from build123d import *

# Parameters (mm, degrees)
F0_T = -12.7
F1_R = 5.08


with BuildPart() as f3:
    # F2 (on Front) → F3 (revolve)
    with BuildSketch(Plane.XZ):
        Polygon((42.4395352602, 50.6010726094), (0, 50.6010726094), (0, -51.2385219336), (24.419054389, -51.2385219336), align=None)
    revolve(axis=Axis((0, 0, -0.3187246621), (0, 0, 1)))

    # F0
    f0_openings = [f3.faces().sort_by_distance(p)[0] for p in [
        (0, 0, 50.601073),
    ]]
    offset(amount=F0_T, openings=f0_openings)

    # F1
    f1_edges = [f3.edges().sort_by_distance(p)[0] for p in [
        (-42.439535, 0, 50.601073),
        (-29.542242, 0, 50.601073),
    ]]
    fillet(f1_edges, radius=F1_R)


solid = f3.part
Here's how the part is built. I have some questions about the finished solid (model axes, mm). Round coordinates to 2 decimals unless told otherwise and drop trailing zeros. Loops run counter-clockwise (first coordinate to the right, second up) from the corner with the lowest first, then second, coordinate; pieces in that order, holes last.
1. If we section it at D-D on z = -45: Write out the boundary of the cut face in (x, y).
Answer list:
outline: circle Ø51.05 at (0, 0)
2. If I drill on line 1 along Z through (x, y) = (-8, 0.5); line 2 along Y through (x, z) = (18.5, 37); line 3 along Y through (x, z) = (14.5, 17.5), over which ranges is the centre line in solid material (lowest first)?
Answer list:
line 1: z = -51.24 to -38.54
line 2: y = -35.5 to -19.85, 19.85 to 35.5
line 3: y = -33.59 to -18.73, 18.73 to 33.59
3. We'd pull the mould along Y, two halves only. Please class faces 1 (the face through (0, 0, -38.539)), 2 (the face through (24.1, -24.1, 50.601)), 3 (the face through (29.7, 9.35, -13.28)): +Y half, -Y half, draft (parallel to the pull), parting line (faces both ways), or undercut.
Answer list:
face 1: undercut
face 2: draft
face 3: parting line
4. For P1, Ø1.5, axis at x = 20, z = 8.5, coming from the -Y side; P2, Ø6, axis at x = -19.5, z = 22.5, coming from the +Y side; P3, Ø10, axis at y = 29, z = -11, coming from the +X side, each with a flat end and sliding along its axis, tell me the tip position at first contact or that it passes through.
Answer list:
P1: stops at y = -29.24
P2: stops at y = 33.75
P3: stops at x = 20.62
5. If we section it at C-C on z = 37.5: Write out the boundary of the cut face in (x, y), plus the area to 3 significant figures.
Answer list:
outline: circle Ø80.24 at (0, 0); hole circle Ø54.45 at (0, 0)
area: 2,730 mm2
6. If we section it at A-A on x = 0: Write out the boundary of the cut face in (y, z).
Answer list:
outline: (-41.38, 44.64) - (-24.42, -51.24) - (24.42, -51.24) - (41.38, 44.64) arc R5.08 ccw to (36.38, 50.6) - (33.8, 50.6) arc R5.08 ccw to (28.8, 46.41) - (13.77, -38.54) - (-13.77, -38.54) - (-28.8, 46.41) arc R5.08 ccw to (-33.8, 50.6) - (-36.38, 50.6) arc R5.08 ccw to start
